CAD build for the part. Positions are in the model's coordinates, mm. A direction names the side the tool comes from. Coordinates: 2 decimals unless noted, no trailing zeros. Write each loop counter-clockwise with the first axis right and the second up, starting at its lowest first coordinate (ties: lowest second). Pieces come first, ordered by that corner, then holes. Notation, with made-up numbers: (62.5, 1) - (114.5, 1) arc R28 ccw to (114.5, 33) - close; hole circle Ø11 at (45.25, 79.5). An arc over 180 degrees is marked (long way). Answer in a Markdown table with one row per item. Add a question column.
Q1. Drill centre lines: line 1 along Z through (x, y) = (-1, -1); line 2 along X through (y, z) = (-0.5, -2.5); line 3 along Z through (x, y) = (2.5, 2.5). Where is each one in solid material? Low to high. Write a range as from..to.
Q2. Band-saw the part on C-C (z = -23). List the corners of the cut face in (x, y).
Q3. Band-saw the part on B-B (x = 0). List the corners of the cut face in (y, z).
Q4. Band-saw the part on A-A (y = 0). List the corners of the cut face in (x, z), and give its area (3 significant figures).
Q5. Pin check, flat tips, straight feed: pin 1 (2 mm diameter, centred on y = -3, z = -0.5, fed in from -X); pin 2 (4 mm diameter, centred on x = 1.5, z = -1.5, fed in from +Y); pin 3 (1.5 mm diameter, centred on x = -2, z = -16, fed in from +Y). Stop position of each tip, or through.
Q6. Band-saw the part on D-D (y = 2). List the corners of the cut face in (x, z), and give its area (3 significant figures).
Q7. 3-axis set-ups, long thin cutter, end or side, ignore diameter. For faces 1 (the flat face through (-1, 3, 0)), 2 (the flat face through (0, 0, 2.5)), 3 (the flat face through (0, 1, -20)), 4 (the cylindrical face through (-0.802, 3.612, 1.232)), 5 (the cylindrical face through (0, 1.5, -20.2)): which of +Z, -Z, +X, -X, +Y, -Y reach the whole face in a straight line?
Autodesk Fusion 360 part; units mm, degrees
sketch "Sketch1" plane through (0, 0, 0) normal (0, 0, 1) x (1, 0, 0)
  circle A0 centre (0, 0) radius 3
  circle A1 centre (0, 0) radius 3.7
  dimension "d1" = 6
  dimension "d2" = 7.4
extrude "Extrude1" add sketch "Sketch1" along normal blind 2.5 contours A0 | A1
extrude "Extrude2" add sketch "Sketch1" against normal blind 15.8 contours A0
sketch "Sketch2" plane through (0, 0, -15.8) normal (0, 0, -1) x (-1, 0, 0)
  circle A0 centre (0, 0) radius 3
  circle A1 centre (0, 0) radius 1.5
  line L0 (-2.2147, 1) -> (2, 1)
  dimension "d7" = 3
  dimension "d8" = 1
extrude "Extrude3" add sketch "Sketch2" along normal blind 9 contours A1 L0 picked at (-0.0369, 1.2519)
Checked values:
| question | item | result |
|---|---|---|
| 1 | line 1 | z = -15.8..2.5 |
| 1 | line 2 | x = -2.96..2.96 |
| 1 | line 3 | z = 0..2.5 |
| 2 | outline | (-1.12, 1) - (1.12, 1) arc R1.5 ccw to start |
| 3 | outline | (-3.7, 0) - (-3, 0) - (-3, -15.8) - (1, -15.8) - (1, -24.8) - (1.5, -24.8) - (1.5, -15.8) - (3, -15.8) - (3, 0) - (3.7, 0) - (3.7, 2.5) - (-3.7, 2.5) - close |
| 4 | outline | (-3.7, 0) - (-3, 0) - (-3, -15.8) - (3, -15.8) - (3, 0) - (3.7, 0) - (3.7, 2.5) - (-3.7, 2.5) - close |
| 4 | area | 113 mm² |
| 5 | pin 1 | stops at x = -3.02 |
| 5 | pin 2 | stops at y = 3.7 |
| 5 | pin 3 | stops at y = 2.71 |
| 6 | outline | (-3.11, 0) - (-2.24, 0) - (-2.24, -15.8) - (2.24, -15.8) - (2.24, 0) - (3.11, 0) - (3.11, 2.5) - (-3.11, 2.5) - close |
| 6 | area | 86.2 mm² |
| 7 | face 1 | -Z |
| 7 | face 2 | +Z, +X, -X, +Y, -Y |
| 7 | face 3 | -Z, +X, -X, -Y |
| 7 | face 4 | +Z, -Z |
| 7 | face 5 | -Z, +Y |
